```python
from build123d import *

# Parameters (mm, degrees)
F0_R     = 0.625
F0_R_2   = 0.5
F1_DEPTH = 4
F2_W     = 1.5
F2_H     = 0.5
F3_DEPTH = 1


with BuildPart() as f1:
    # F0 (on Right) → F1 (new body, symmetric)
    with BuildSketch(Plane.YZ):
        with Locations((-0.079547, 0)):
            Circle(F0_R)
        with Locations((-0.079547, 0)):
            Circle(F0_R_2, mode=Mode.SUBTRACT)
    extrude(amount=F1_DEPTH, both=True)

    # F2 (on Front) → F3 (cut, symmetric)
    with BuildSketch(Plane.XZ):
        with Locations((0, 0.590535)):
            Rectangle(F2_W, F2_H)
    extrude(amount=F3_DEPTH, both=True, mode=Mode.SUBTRACT)


solid = f1.part
```
Geometry: final body of the model. Coordinates: model frame, mm. Give positions to 0.01 mm unless a question says otherwise; leave off trailing zeros. Write each loop counter-clockwise with the first axis right and the second up, starting at its lowest first coordinate (ties: lowest second). Pieces come first, ordered by that corner, then holes.
1. Section query B-B, the plane y = -0.1. Return loops of the section in (x, z).
2. Section query D-D, the plane z = -0.35. Return loops of the section in (x, y), then the cut area to 3 significant figures.
3. Section query C-C, the plane x = 2. Return loops of the section in (y, z) (3 decimals), then the cut area to 3 significant figures.
4. Line query: probe 1 along X at (y, z) = (0.15, 0.5); probe 2 along Y at (x, z) = (-3.5, -0.35). Output: solid intervals per line, ascending.
5. Section query A-A, the plane z = 0. Return loops of the section in (x, y), then the cut area to 3 significant figures.
Computed:
1. outline: (-4, -0.62) - (4, -0.62) - (4, -0.5) - (-4, -0.5) - close; (-4, 0.5) - (-0.75, 0.5) - (-0.75, 0.62) - (-4, 0.62) - close; (0.75, 0.5) - (4, 0.5) - (4, 0.62) - (0.75, 0.62) - close
2. outline: (-4, -0.6) - (4, -0.6) - (4, -0.44) - (-4, -0.44) - close; (-4, 0.28) - (4, 0.28) - (4, 0.44) - (-4, 0.44) - close
2. area: 2.57 mm2
3. outline: circle Ø1.25 at (-0.08, 0); hole circle Ø1 at (-0.08, 0)
3. area: 0.442 mm2
4. probe 1: x = -4 to -0.75, 0.75 to 4
4. probe 2: y = -0.6 to -0.44, 0.28 to 0.44
5. outline: (-4, -0.7) - (4, -0.7) - (4, -0.58) - (-4, -0.58) - close; (-4, 0.42) - (4, 0.42) - (4, 0.55) - (-4, 0.55) - close
5. area: 2.00 mm2
